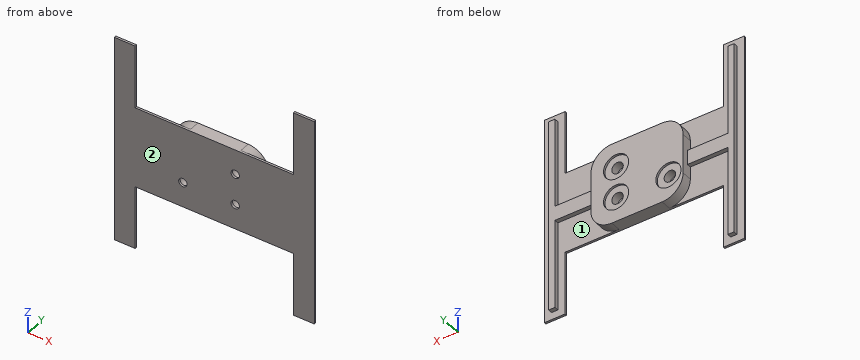
```python
from build123d import *

# Parameters (mm, degrees)
SKETCH1_R           = 1.75
BOSS_EXTRUDE1_DEPTH = 6
SKETCH2_R           = 2.75
CUT_EXTRUDE1_DEPTH  = 5
SKETCH3_R           = 6
CUT_EXTRUDE2_DEPTH  = 1
BOSS_EXTRUDE3_DEPTH = 1
BOSS_EXTRUDE4_DEPTH = 2
SKETCH7_R           = 2
CUT_EXTRUDE3_DEPTH  = 2


with BuildPart() as part:
    # Sketch1 → Boss-Extrude1 (new body)
    with BuildSketch(Plane(origin=(0, 0, 0), x_dir=(1, 0, 0), z_dir=(0, 1, 0))):
        with BuildLine():
            Line((-11.011362906, -24.58650519), (12.988637094, -24.58650519))
            ThreePointArc((12.988637094, -24.58650519), (20.059704906, -21.657573002), (22.988637094, -14.58650519))
            Line((22.988637094, -14.58650519), (22.988637094, 4.41349481))
            ThreePointArc((22.988637094, 4.41349481), (20.059704906, 11.484562622), (12.988637094, 14.41349481))
            Line((12.988637094, 14.41349481), (-11.011362906, 14.41349481))
            ThreePointArc((-11.011362906, 14.41349481), (-18.082430717, 11.484562622), (-21.011362906, 4.41349481))
            Line((-21.011362906, 4.41349481), (-21.011362906, -14.58650519))
            ThreePointArc((-21.011362906, -14.58650519), (-18.082430717, -21.657573002), (-11.011362906, -24.58650519))
        make_face()
        with Locations((-14.011362906, 2.41349481)):
            Circle(SKETCH1_R, mode=Mode.SUBTRACT)
        with Locations((10.988637094, 2.41349481)):
            Circle(SKETCH1_R, mode=Mode.SUBTRACT)
        with Locations((10.988637094, -12.58650519)):
            Circle(SKETCH1_R, mode=Mode.SUBTRACT)
    extrude(amount=BOSS_EXTRUDE1_DEPTH)

    # Sketch2 → Cut-Extrude1 (cut)
    with BuildSketch(Plane(origin=(0, 6, 0), x_dir=(1, 0, 0), z_dir=(0, 1, 0))):
        with Locations((-14.011362906, 2.41349481)):
            Circle(SKETCH2_R)
        with Locations((10.988637094, 2.41349481)):
            Circle(SKETCH2_R)
        with Locations((10.988637094, -12.58650519)):
            Circle(SKETCH2_R)
    extrude(amount=-CUT_EXTRUDE1_DEPTH, mode=Mode.SUBTRACT)

    # Sketch3 → Cut-Extrude2 (cut)
    with BuildSketch(Plane(origin=(0, 6, 0), x_dir=(1, 0, 0), z_dir=(0, 1, 0))):
        with Locations((10.988637094, 2.41349481)):
            Circle(SKETCH3_R)
        with Locations((10.988637094, -12.58650519)):
            Circle(SKETCH3_R)
        with Locations((-14.011362906, 2.41349481)):
            Circle(SKETCH3_R)
    extrude(amount=-CUT_EXTRUDE2_DEPTH, mode=Mode.SUBTRACT)

    # Sketch4 → Boss-Extrude3 (add)
    with BuildSketch(Plane.XZ):
        Polygon((-46.776393851, -44.91349481), (-36.776393851, -44.91349481), (-36.776393851, -14.41349481), (38.75366804, -14.41349481), (38.75366804, -44.91349481), (48.75366804, -44.91349481), (48.75366804, 55.08650519), (38.75366804, 55.08650519), (38.75366804, 24.58650519), (-36.776393851, 24.58650519), (-36.776393851, 55.08650519), (-46.776393851, 55.08650519), align=None)
    extrude(amount=-BOSS_EXTRUDE3_DEPTH)

    # Sketch6 → Boss-Extrude4 (add)
    with BuildSketch(Plane(origin=(0, 1, 0), x_dir=(1, 0, 0), z_dir=(0, 1, 0))):
        Polygon((22.988637094, -1.58650519), (42.25366804, -1.58650519), (42.25366804, 41.4051813), (45.25366804, 41.4051813), (45.25366804, -51.58650519), (42.25366804, -51.58650519), (42.25366804, -8.58650519), (22.988637094, -8.58650519), align=None)
        Polygon((-21.011362906, -8.58650519), (-21.011362906, -1.58650519), (-40.276393851, -1.58650519), (-40.276393851, 41.4051813), (-43.276393851, 41.4051813), (-43.276393851, -51.58650519), (-40.276393851, -51.58650519), (-40.276393851, -8.58650519), align=None)
    extrude(amount=BOSS_EXTRUDE4_DEPTH)

    # Sketch7 → Cut-Extrude3 (cut)
    with BuildSketch(Plane.XZ):
        with Locations((-14.011362906, -2.41349481)):
            Circle(SKETCH7_R)
        with Locations((10.988637094, -2.41349481)):
            Circle(SKETCH7_R)
        with Locations((10.988637094, 12.58650519)):
            Circle(SKETCH7_R)
    extrude(amount=-CUT_EXTRUDE3_DEPTH, mode=Mode.SUBTRACT)


solid = part.part
```
Could you check a few things on this model? Use its own coordinates, in mm. Face numbers are marked on the shaded views. Round coordinates to 2 decimals unless told otherwise and drop trailing zeros. Loops run counter-clockwise (first coordinate to the right, second up) from the corner with the lowest first, then second, coordinate; pieces in that order, holes last.
Q1. I want a section at A-A (z = 43). Write out the boundary of the cut face in (x, y).
Q2. I want a section at D-D (x = -24). Write out the boundary of the cut face in (y, z).
Q3. Please list where these lines run through material, in increasing order: L1, parallel to Z at x = 12.5, y = 3.35; L2, parallel to X at y = 1.95, z = 14; L3, parallel to X at y = 1.8, z = 25.5.
Q4. I want a section at C-C (y = 2.1). Write out the boundary of the cut face in (x, z), and give its area (3 significant figures).
Q5. I want a section at B-B (x = -14). Write out the boundary of the cut face in (y, z).
Q6. For P1, Ø2, axis at x = -29.5, z = 11.5, coming from the +Y side; P2, Ø2.5, axis at x = 10.99, z = 12.59, coming from the -Y side; P3, Ø1, axis at x = -41.5, y = 2.5, coming from the -Z side; P4, Ø1.6, axis at y = 2.5, z = -26.5, coming from the +X side, each with a flat end and sliding along its axis, tell me the tip position at first contact or that it passes through.
Q7. Thinking about a two-plate mould opening in X: for the marked faces 1 and 2, which applies, pulls with the +X half, pulls with the -X half, needs draft (parallel to the pull), parting line crosses it, or undercut?
Answer below:
1. outline: (-46.78, 0) - (-36.78, 0) - (-36.78, 1) - (-40.28, 1) - (-40.28, 3) - (-43.28, 3) - (-43.28, 1) - (-46.78, 1) - close; (38.75, 0) - (48.75, 0) - (48.75, 1) - (45.25, 1) - (45.25, 3) - (42.25, 3) - (42.25, 1) - (38.75, 1) - close
2. outline: (0, -14.41) - (1, -14.41) - (1, 1.59) - (3, 1.59) - (3, 8.59) - (1, 8.59) - (1, 24.59) - (0, 24.59) - close
3. L1: z = -14.41 to -4.71, -0.12 to 10.29, 14.88 to 24.59
3. L2: x = -43.28 to -40.28, -21.01 to 8.63, 13.35 to 22.99, 42.25 to 45.25
3. L3: x = -43.28 to -40.28, 42.25 to 45.25
4. outline: (-43.28, -41.41) - (-40.28, -41.41) - (-40.28, 1.59) - (-21.01, 1.59) - (-21.01, -4.41) arc R10 ccw to (-11.01, -14.41) - (12.99, -14.41) arc R10 ccw to (22.99, -4.41) - (22.99, 1.59) - (42.25, 1.59) - (42.25, -41.41) - (45.25, -41.41) - (45.25, 51.59) - (42.25, 51.59) - (42.25, 8.59) - (22.99, 8.59) - (22.99, 14.59) arc R10 ccw to (12.99, 24.59) - (-11.01, 24.59) arc R10 ccw to (-21.01, 14.59) - (-21.01, 8.59) - (-40.28, 8.59) - (-40.28, 51.59) - (-43.28, 51.59) - close; hole circle Ø5.5 at (-14.01, -2.41); hole circle Ø5.5 at (10.99, -2.41); hole circle Ø5.5 at (10.99, 12.59)
4. area: 2,390 mm2
5. outline: (0, -14.41) - (1, -14.41) - (1, -13.96) - (6, -13.96) - (6, -8.41) - (5, -8.41) - (5, -5.16) - (1, -5.16) - (1, -4.41) - (0, -4.41) - close; (0, -0.41) - (1, -0.41) - (1, 0.34) - (5, 0.34) - (5, 3.59) - (6, 3.59) - (6, 24.13) - (1, 24.13) - (1, 24.59) - (0, 24.59) - close
6. P1: stops at y = 1
6. P2: passes through
6. P3: stops at z = -41.41
6. P4: stops at x = 45.25
7. face 1: undercut
7. face 2: needs draft
